```python
from build123d import *

# Parameters (mm, degrees)
SKETCH1_R           = 1.65
BOSS_EXTRUDE1_DEPTH = 3
SKETCH3_W           = 11
SKETCH3_H           = 6
CUT_EXTRUDE2_DEPTH  = 1.2
SKETCH4_R           = 1.65
BOSS_EXTRUDE2_DEPTH = 1.2


with BuildPart() as part:
    # Sketch1 → Boss-Extrude1 (new body)
    with BuildSketch(Plane(origin=(0, 0, 0), x_dir=(0, 0, -1), z_dir=(1, 0, 0))):
        with BuildLine():
            Line((0, 3), (40.5, 3))
            ThreePointArc((40.5, 3), (43.5, 0), (40.5, -3))
            Line((40.5, -3), (0, -3))
            ThreePointArc((0, -3), (-3, 0), (0, 3))
        make_face()
        Circle(SKETCH1_R, mode=Mode.SUBTRACT)
        with Locations((40.5, 0)):
            Circle(SKETCH1_R, mode=Mode.SUBTRACT)
    extrude(amount=BOSS_EXTRUDE1_DEPTH)

    # Sketch3 → Cut-Extrude2 (cut)
    with BuildSketch(Plane.ZY):
        with Locations((-38, 0)):
            Rectangle(SKETCH3_W, SKETCH3_H)
    extrude(amount=-CUT_EXTRUDE2_DEPTH, mode=Mode.SUBTRACT)

    # Sketch4 → Boss-Extrude2 (add)
    with BuildSketch(Plane(origin=(3, 0, 0), x_dir=(0, 0, -1), z_dir=(1, 0, 0))):
        with BuildLine():
            Line((40.5, 3), (23.5, 3))
            Line((23.5, 3), (23.5, -3))
            Line((23.5, -3), (40.5, -3))
            ThreePointArc((40.5, -3), (43.5, 0), (40.5, 3))
        make_face()
        with Locations((40.5, 0)):
            Circle(SKETCH4_R, mode=Mode.SUBTRACT)
    extrude(amount=BOSS_EXTRUDE2_DEPTH)


solid = part.part
```
Check sheet for the modelled part. Datum: model origin and axes. Units: mm. A direction names the side the tool comes from. Coordinates: 2 decimals unless noted, no trailing zeros. Write each loop counter-clockwise with the first axis right and the second up, starting at its lowest first coordinate (ties: lowest second). Pieces come first, ordered by that corner, then holes. Notation, with made-up numbers: (32, 40) - (65, 40) arc R29 ccw to (65, 74) - close; hole circle Ø8 at (-14, 87.25). An arc over 180 degrees is marked (long way). One line per question, with ' | ' between items.
Item 1: Sectioned sample at B-B on y = -2.4. Record the boundary of the cut face in (x, z), plus the area to 3 significant figures.
Determined:
outline: (0, -32.5) - (1.2, -32.5) - (1.2, -42.3) - (4.2, -42.3) - (4.2, -23.5) - (3, -23.5) - (3, 1.8) - (0, 1.8) - close | area: 143 mm2
Item 2: Access from +Z, -Z, +X, -X, +Y, -Y to the whole of each face (thin tool, end or side, straight path). Record for faces 1 (the face through (1.2, 0, -37)), 2 (the face through (2, -3, -20)).
Determined:
face 1: -Z, -X, +Y, -Y | face 2: +Z, -Z, +X, -X, -Y
Item 3: Thickness scan on line 1 (Y direction, x = 3.35, z = -40.5); line 2 (Z direction, x = 1.5, y = 0.6); line 3 (X direction, y = -1.45, z = -9.5). Record the ranges inside material, lowest first. Write a range as [from, to].
Determined:
line 1: y = [-3, -1.65], [1.65, 3] | line 2: z = [-43.44, -42.04], [-38.96, -1.54], [1.54, 2.94] | line 3: x = [0, 3]
Item 4: Sectioned sample at C-C on z = -15.5. Record the boundary of the cut face in (x, y).
Determined:
outline: (0, -3) - (3, -3) - (3, 3) - (0, 3) - close
Item 5: Mould release check, pull along Z, two halves, no side actions. Record for faces 3 (the face through (3, 0, -10)), 4 (the face through (4, 0, -23.5)), 5 (the face through (1.479, 1.115, 1.216)): pulls with the +Z half, pulls with the -Z half, needs draft (parallel to the pull), parting line crosses it, or undercut.
Determined:
face 3: needs draft | face 4: pulls with the +Z half | face 5: undercut
Item 6: Sectioned sample at A-A on y = 0.8. Record the boundary of the cut face in (x, z), plus the area to 3 significant figures.
Determined:
outline: (0, -32.5) - (1.2, -32.5) - (1.2, -39.06) - (4.2, -39.06) - (4.2, -23.5) - (3, -23.5) - (3, -1.44) - (0, -1.44) - close; (0, 1.44) - (3, 1.44) - (3, 2.89) - (0, 2.89) - close; (1.2, -43.39) - (4.2, -43.39) - (4.2, -41.94) - (1.2, -41.94) - close | area: 132 mm2
Item 7: Gauge pin test, flat ends, axial feed: P1, Ø1.5, axis at x = 1, y = -1.5, coming from the -Z side; P2, Ø1, axis at x = 2.5, y = 1.5, coming from the -Z side. Record the tip position at first contact, or that the pin passes through.
Determined:
P1: stops at z = -43.4 | P2: stops at z = -43.33
